CAD build for the part. Positions are in the model's coordinates, mm. A direction names the side the tool comes from. Round coordinates to 2 decimals unless told otherwise and drop trailing zeros. Write each loop counter-clockwise with the first axis right and the second up, starting at its lowest first coordinate (ties: lowest second). Pieces come first, ordered by that corner, then holes. Notation, with made-up numbers: (40.25, 25) -> (79.25, 25) arc R25 cw to (79.25, 55) -> close; hole circle Ø6 at (80.25, 47). An arc over 180 degrees is marked (long way). Answer in a Markdown table with one row per item. Add a question column.
```python
from build123d import *

# Parameters (mm, degrees)
F0_R          = 8.875
F1_DEPTH      = 4
F1_DEPTH_BACK = 4
F2_SIZE       = 1
F3_DEPTH      = 4
F3_DEPTH_BACK = 4
F4_DEPTH      = 0.5
F4_DEPTH_BACK = 0.5


with BuildPart() as f1:
    # F0 (on Front) → F1 (new body, two sides)
    with BuildSketch(Plane.XZ) as f1_sk:
        with BuildLine():
            ThreePointArc((-10.375, 0), (0, -10.375), (10.375, 0))
            ThreePointArc((10.375, 0), (0, 10.375), (-10.375, 0))
        make_face()
        Circle(F0_R, mode=Mode.SUBTRACT)
    extrude(amount=F1_DEPTH)
    extrude(f1_sk.sketch, amount=-F1_DEPTH_BACK)

    # F2
    f2_edges = [f1.edges().sort_by_distance(p)[0] for p in [
        (-8.875, -4, 0),
        (-8.875, 4, 0),
    ]]
    chamfer(f2_edges, length=F2_SIZE)

    # F0 (on Front) → F3 (join, two sides)
    with BuildSketch(Plane.XZ) as f3_sk:
        with BuildLine():
            ThreePointArc((-10.375, 0), (0, 10.375), (10.375, 0))
            Line((10.375, 0), (10.375, 16.363068172))
            ThreePointArc((10.375, 16.363068172), (0, 19.375), (-10.375, 16.363068172))
            Line((-10.375, 16.363068172), (-10.375, 0))
        make_face()
        with BuildLine():
            ThreePointArc((-10.375, 16.363068172), (0, 19.375), (10.375, 16.363068172))
            Line((10.375, 16.363068172), (10.375, 17.5356779168))
            ThreePointArc((10.375, 17.5356779168), (0, 20.375), (-10.375, 17.5356779168))
            Line((-10.375, 17.5356779168), (-10.375, 16.363068172))
        make_face()
    extrude(amount=F3_DEPTH)
    extrude(f3_sk.sketch, amount=-F3_DEPTH_BACK)

    # F0 (on Front) → F4 (cut, two sides)
    with BuildSketch(Plane.XZ) as f4_sk:
        with BuildLine():
            ThreePointArc((-10.375, 16.363068172), (0, 19.375), (10.375, 16.363068172))
            Line((10.375, 16.363068172), (10.375, 17.5356779168))
            ThreePointArc((10.375, 17.5356779168), (0, 20.375), (-10.375, 17.5356779168))
            Line((-10.375, 17.5356779168), (-10.375, 16.363068172))
        make_face()
    extrude(amount=-F4_DEPTH, mode=Mode.SUBTRACT)
    extrude(f4_sk.sketch, amount=F4_DEPTH_BACK, mode=Mode.SUBTRACT)


solid = f1.part
```
Item 1: Drill centre lines: probe 1 along Z at (x, y) = (0, -0.3) (3 decimals); probe 2 along Y at (x, z) = (-5.25, 19.5); probe 3 along X at (y, z) = (-1, -3). Where is each one in solid material? Low to high.
Item 2: Tool access for faces 1 (the cylindrical face through (-1.924, 0.042, -8.664)), 2 (the flat face through (-1, 0.5, 20)): list every direction of +Z, -Z, +X, -X, +Y, -Y with a clear straight run to the whole face (end or side of a thin tool).
Item 3: Pin check, flat tips, straight feed: pin 1 (2 mm diameter, centred on y = -2.5, z = -3.5, fed in from -X); pin 2 (3 mm diameter, centred on y = 2.5, z = -4.5, fed in from -X); pin 3 (8 mm diameter, centred on x = 5.5, z = 0, fed in from +Y) (3 decimals). Stop position of each tip, or through.
Item 4: Two-plate mould, pull along Y, no slides. Class faces 3 (the flat face through (0, -4, 12)), 4 (the flat face through (0, 4, 12)), 5 (the flat face through (-1, -0.5, 20)): +Y half, -Y half, draft (parallel to the pull), parting line (faces both ways), or undercut.
Item 5: Saw through at A-A on x = 0. Give the cut face in (y, z) (3 decimals).
Recorded:
| question | item | result |
|---|---|---|
| 1 | probe 1 | -10.375 to -8.875, 8.875 to 19.375 |
| 1 | probe 2 | -4 to -0.5, 0.5 to 4 |
| 1 | probe 3 | -9.93 to -8.35, 8.35 to 9.93 |
| 2 | face 1 | +Y, -Y |
| 2 | face 2 | +Z |
| 3 | pin 1 | x = -10.07 |
| 3 | pin 2 | x = -9.93 |
| 3 | pin 3 | y = 3.625 |
| 4 | face 3 | -Y half |
| 4 | face 4 | +Y half |
| 4 | face 5 | undercut |
| 5 | outline | (-4, -10.375) -> (4, -10.375) -> (4, -9.875) -> (3, -8.875) -> (-3, -8.875) -> (-4, -9.875) -> close; (-4, 9.875) -> (-3, 8.875) -> (3, 8.875) -> (4, 9.875) -> (4, 20.375) -> (0.5, 20.375) -> (0.5, 19.375) -> (-0.5, 19.375) -> (-0.5, 20.375) -> (-4, 20.375) -> close |
